```python
from build123d import *

# Parameters (mm, degrees)
SKETCH1_R                            = 25
BOSS_EXTRUDE1_DEPTH                  = 100
SKETCH7_R                            = 12.5
THRU_HOLE_DEPTH                      = 107.066017178
SKETCH5_W                            = 5
SKETCH5_H                            = 25
MOUNT_FLATS_DEPTH                    = 107.066017178
F_10_32_TAPPED_HOLE3_D               = 4.0386
F_10_32_TAPPED_HOLE3_DEPTH           = 30
F_10_32_TAPPED_HOLE3_TIP             = 1.213317848
SKETCH6_W                            = 20
SKETCH6_H                            = 40
WINDOW_SLOT_1_DEPTH                  = 106.61249926
WINDOW_SLOT_2_DEPTH                  = 106.61249926
WINDOW_SLOT_2_DEPTH_BACK             = 106.61249926
SKETCH18_W                           = 22.5
SKETCH18_H                           = 40
F_10_32_TAPPED_HOLE2_D               = 4.0386
F_10_32_TAPPED_HOLE2_DEPTH           = 9
F_10_32_TAPPED_HOLE2_TIP             = 1.213317848
F_10_32_TAPPED_HOLE2_ON_FACE_2_D     = 4.0386
F_10_32_TAPPED_HOLE2_ON_FACE_2_DEPTH = 9
F_10_32_TAPPED_HOLE2_ON_FACE_2_TIP   = 1.213317848
SKETCH22_R                           = 2.5273
SKETCH22_R_2                         = 12.5
BOSS_EXTRUDE2_DEPTH                  = 6.35
SAVE_START                           = 100
SAVE_BODIES2_OUTLINE_R               = 2.5273
SAVE_BODIES2_OUTLINE_R_2             = 12.5
SAVE_BODIES2_DEPTH                   = 6.35


# Read off the part's stored shape, not the designer's step: Save Bodies2
with BuildPart() as part:
    # Sketch1 → Boss-Extrude1 (new body)
    with BuildSketch(Plane(origin=(0, 0, 0), x_dir=(1, 0, 0), z_dir=(0, 1, 0))):
        with Locations(Location((0, 0, 0), (0, 0, 270))):
            Circle(SKETCH1_R)
    extrude(amount=BOSS_EXTRUDE1_DEPTH)

    # Sketch7 → Thru Hole (cut, through all)
    with BuildSketch(Plane(origin=(0, 0, 0), x_dir=(1, 0, 0), z_dir=(0, 1, 0))):
        with Locations(Location((0, 0, 0), (0, 0, 270))):
            Circle(SKETCH7_R)
    extrude(amount=THRU_HOLE_DEPTH, mode=Mode.SUBTRACT)

    # Sketch5 → Mount Flats (cut, through all)
    with BuildSketch(Plane(origin=(0, 0, 0), x_dir=(1, 0, 0), z_dir=(0, 1, 0))):
        with Locations((-25.5, 0)):
            Rectangle(SKETCH5_W, SKETCH5_H)
        with Locations((25.5, 0)):
            Rectangle(SKETCH5_W, SKETCH5_H)
    extrude(amount=MOUNT_FLATS_DEPTH, mode=Mode.SUBTRACT)

    # #10-32 Tapped Hole3
    with Locations(Plane(origin=(0, 100, 0), x_dir=(1, 0, 0), z_dir=(0, 1, 0))):
        with Locations((0, 18.75), (-18.75, 0), (0, -18.75), (18.75, 0)):
            Hole(F_10_32_TAPPED_HOLE3_D / 2, depth=F_10_32_TAPPED_HOLE3_DEPTH)
            with Locations((0, 0, -(F_10_32_TAPPED_HOLE3_DEPTH + F_10_32_TAPPED_HOLE3_TIP / 2))):  # 118° drill point
                Cone(0, F_10_32_TAPPED_HOLE3_D / 2, F_10_32_TAPPED_HOLE3_TIP, mode=Mode.SUBTRACT)

    # Sketch6 → Window Slot 1 (cut, symmetric)
    with BuildSketch(Plane(origin=(0, 0, 0), x_dir=(0, 0, -1), z_dir=(1, 0, 0))):
        with Locations((19.797958971, 30)):
            Rectangle(SKETCH6_W, SKETCH6_H)
    window_slot_1 = extrude(amount=WINDOW_SLOT_1_DEPTH, both=True, mode=Mode.SUBTRACT)

    # Mirror2: Window Slot 1 across plane
    add(window_slot_1.mirror(Plane.XY), mode=Mode.SUBTRACT)

    # Sketch18 → Window Slot 2 (cut, two sides: drawn at the far end of the back side and taken through both)
    with BuildSketch(Plane.XY.offset(-WINDOW_SLOT_2_DEPTH_BACK)):
        with Locations((0, 30)):
            Rectangle(SKETCH18_W, SKETCH18_H)
    extrude(amount=WINDOW_SLOT_2_DEPTH + WINDOW_SLOT_2_DEPTH_BACK, mode=Mode.SUBTRACT)

    # #10-32 Tapped Hole2
    with Locations(Plane(origin=(-23, 60, 5), x_dir=(0, 0, -1), z_dir=(-1, 0, 0))):
        with Locations((0, 0), (10, 0)):
            Hole(F_10_32_TAPPED_HOLE2_D / 2, depth=F_10_32_TAPPED_HOLE2_DEPTH)
            with Locations((0, 0, -(F_10_32_TAPPED_HOLE2_DEPTH + F_10_32_TAPPED_HOLE2_TIP / 2))):  # 118° drill point
                Cone(0, F_10_32_TAPPED_HOLE2_D / 2, F_10_32_TAPPED_HOLE2_TIP, mode=Mode.SUBTRACT)

    # #10-32 Tapped Hole2 on face 2
    with Locations(Plane(origin=(23, 60, 5), x_dir=(0, 0, 1), z_dir=(1, 0, 0))):
        with Locations((0, 0), (-10, 0)):
            Hole(F_10_32_TAPPED_HOLE2_ON_FACE_2_D / 2, depth=F_10_32_TAPPED_HOLE2_ON_FACE_2_DEPTH)
            with Locations((0, 0, -(F_10_32_TAPPED_HOLE2_ON_FACE_2_DEPTH + F_10_32_TAPPED_HOLE2_ON_FACE_2_TIP / 2))):  # 118° drill point
                Cone(0, F_10_32_TAPPED_HOLE2_ON_FACE_2_D / 2, F_10_32_TAPPED_HOLE2_ON_FACE_2_TIP, mode=Mode.SUBTRACT)


with BuildPart() as body_2:
    # Sketch22 → Boss-Extrude2 (new body)
    with BuildSketch(Plane(origin=(0, 100, 0), x_dir=(1, 0, 0), z_dir=(0, 1, 0))):
        with BuildLine():
            Line((23, -9.797958971), (23, 9.797958971))
            ThreePointArc((23, 9.797958971), (0, 25), (-23, 9.797958971))
            Line((-23, 9.797958971), (-23, -9.797958971))
            ThreePointArc((-23, -9.797958971), (0, -25), (23, -9.797958971))
        make_face()
        with Locations(Location((-18.75, 0, 0), (0, 0, 270))):
            Circle(SKETCH22_R, mode=Mode.SUBTRACT)
        with Locations(Location((0, 18.75, 0), (0, 0, 270))):
            Circle(SKETCH22_R, mode=Mode.SUBTRACT)
        with Locations(Location((18.75, 0, 0), (0, 0, 270))):
            Circle(SKETCH22_R, mode=Mode.SUBTRACT)
        with Locations(Location((0, -18.75, 0), (0, 0, 270))):
            Circle(SKETCH22_R, mode=Mode.SUBTRACT)
        with Locations(Location((0, 0, 0), (0, 0, 270))):
            Circle(SKETCH22_R_2, mode=Mode.SUBTRACT)
    extrude(amount=BOSS_EXTRUDE2_DEPTH)

    # Save Bodies2 outline → Save Bodies2 (cut)
    with BuildSketch(Plane(origin=(0, 0, 0), x_dir=(1, 0, 0), z_dir=(0, 1, 0)).offset(SAVE_START)):
        with BuildLine():
            ThreePointArc((-23, -9.797958971), (0, -25), (23, -9.797958971))
            Line((23, -9.797958971), (23, 9.797958971))
            ThreePointArc((23, 9.797958971), (0, 25), (-23, 9.797958971))
            Line((-23, 9.797958971), (-23, -9.797958971))
        make_face()
        with Locations((0, -18.75)):
            Circle(SAVE_BODIES2_OUTLINE_R, mode=Mode.SUBTRACT)
        with Locations((-18.75, 0)):
            Circle(SAVE_BODIES2_OUTLINE_R, mode=Mode.SUBTRACT)
        Circle(SAVE_BODIES2_OUTLINE_R_2, mode=Mode.SUBTRACT)
        with Locations((18.75, 0)):
            Circle(SAVE_BODIES2_OUTLINE_R, mode=Mode.SUBTRACT)
        with Locations((0, 18.75)):
            Circle(SAVE_BODIES2_OUTLINE_R, mode=Mode.SUBTRACT)
    extrude(amount=SAVE_BODIES2_DEPTH, mode=Mode.SUBTRACT)


solid = part.part
```
Input: part model. Units: mm. Frame: model coordinates. A direction names the side the tool comes from. Give positions to 0.01 mm unless a question says otherwise; leave off trailing zeros. Order: outer loops, then holes, each group sorted by start corner. A loop starts at its lowest first (then second) coordinate and runs counter-clockwise, first axis right, second up. Notation, with made-up numbers: (45, 40.5) -> (99, 40.5) arc R6 cw to (99, 48.5) -> close; hole circle Ø8 at (80.25, 73.5). An arc over 180 degrees is marked (long way). Write each question's results on one line, items separated by ' | '. Start each with the question number.
Item 1: Line query: line 1 (Y direction, x = 10.5, z = 9); line 2 (Z direction, x = 19.5, y = 60); line 3 (Z direction, x = 1.5, y = 92.5). Output: solid intervals per line, ascending.
Item 2: Mould query, pull axis Z, two halves, no side actions, for faces 1 (the conical face through (13, 59.7, 5.19)), 2 (the cylindrical face through (0, 75, 25)), 3 (the flat face through (-11.25, 30, -8)), 4 (the conical face through (-19.1, 68.997, -0.015)). Classes: pulls with the +Z half, pulls with the -Z half, needs draft (parallel to the pull), parting line crosses it, or undercut.
Item 3: Contact query for flat-ended pins moving along their axis: P1, Ø6, axis at x = 18, y = 35.5, coming from the -Z side; P2, Ø5, axis at x = -14, y = 22, coming from the +Z side; P3, Ø3.5, axis at y = 60, z = 5, coming from the -X side. Output: stop coordinate, or through.
Item 4: Cut plane D-D on y = 67. Return the cut outline in (x, z), then the cut area to 3 significant figures.
Item 5: Cut plane B-B on y = 13. Return the cut outline in (x, z), then the cut area to 3 significant figures.
Item 6: Cut plane C-C on x = 6.5. Return the cut outline in (y, z), then the cut area to 3 significant figures.
Item 7: Set-up query: faces 5 (the cylindrical face through (0.44, 84.79, -16.78)), 6 (the cylindrical face through (18.437, 57.998, -4.737)), 7 (the flat face through (11.25, 30, -8)), 8 (the cylindrical face through (-18.437, 57.998, -5.263)). Return all of +Z, -Z, +X, -X, +Y, -Y with unobstructed straight access to the full face (end or side cutting, diameter ignored); none if empty.
Item 8: Cut plane A-A on z = 15. Return the cut outline in (x, y).
Established:
1) line 1: 0 to 10, 50 to 100 | line 2: -15.64 to -7.02, -2.98 to 2.98, 7.02 to 15.64 | line 3: -24.95 to -20.1, -17.4 to -12.41, 12.41 to 17.4, 20.1 to 24.95
2) face 1: undercut | face 2: pulls with the +Z half | face 3: needs draft | face 4: undercut
3) P1: z = -9.8 | P2: z = 9.8 | P3: x = -13.84
4) outline: (-23, -9.8) arc R25 ccw to (23, -9.8) -> (23, 9.8) arc R25 ccw to (-23, 9.8) -> close; hole circle Ø25 at (0, 0) | area: 1,420 mm^2
5) outline: (-23, -9.8) -> (-11.25, -9.8) -> (-11.25, -5.45) arc R12.5 cw to (-11.25, 5.45) -> (-11.25, 9.8) -> (-23, 9.8) -> close; (11.25, -9.8) -> (23, -9.8) -> (23, 9.8) -> (11.25, 9.8) -> (11.25, 5.45) arc R12.5 cw to (11.25, -5.45) -> close | area: 442 mm^2
6) outline: (0, -24.14) -> (10, -24.14) -> (10, -10.68) -> (0, -10.68) -> close; (0, 10.68) -> (10, 10.68) -> (10, 24.14) -> (0, 24.14) -> close; (50, -24.14) -> (100, -24.14) -> (100, -10.68) -> (50, -10.68) -> close; (50, 10.68) -> (100, 10.68) -> (100, 24.14) -> (50, 24.14) -> close | area: 1,620 mm^2
7) face 5: +Y | face 6: +X | face 7: +Z, -Z | face 8: -X
8) outline: (-20, 0) -> (20, 0) -> (20, 10) -> (-20, 10) -> close; (-20, 50) -> (20, 50) -> (20, 100) -> (-20, 100) -> close
